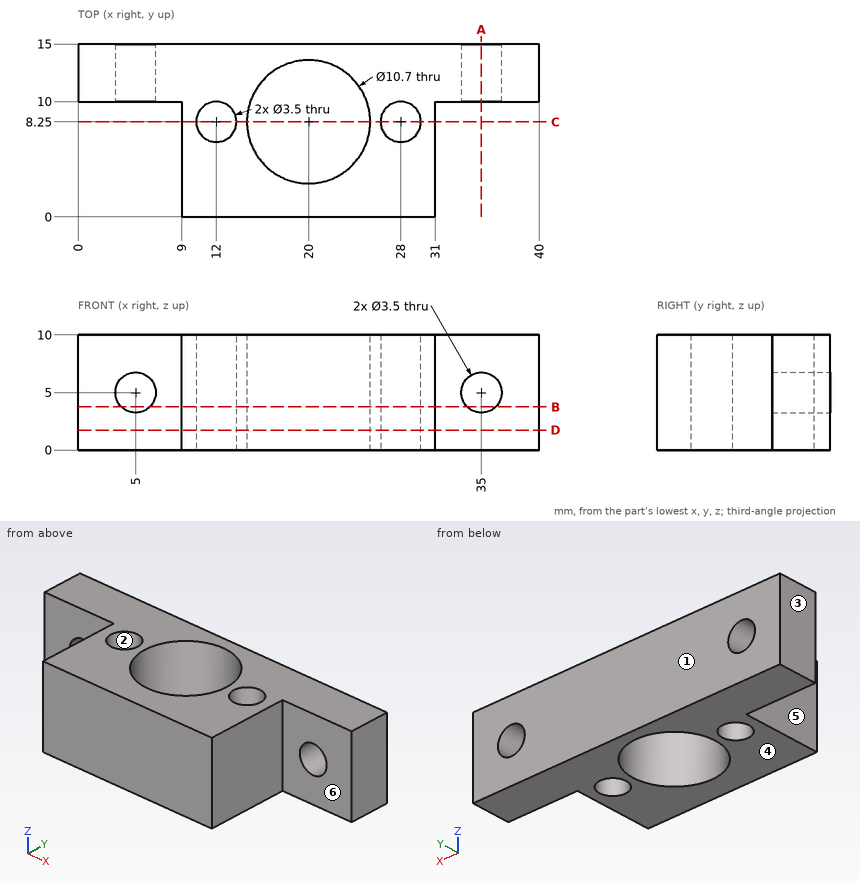
Design review of the part shown in the three views and the two pictorial views. Dimensions are in mm from the part's minimum x, y and z. A direction names the side the tool comes from. Give positions to 0.01 mm unless a question says otherwise; leave off trailing zeros. Write each loop counter-clockwise with the first axis right and the second up, starting at its lowest first coordinate (ties: lowest second). Pieces come first, ordered by that corner, then holes. Notation, with made-up numbers: (-17.75, 30.25) -> (38.25, 30.25) arc R15 ccw to (38.25, 55.25) -> close; hole circle Ø4 at (-8.75, 70). An arc over 180 degrees is marked (long way). Answer in a Markdown table with one row per item.
1) Add section A-A on x = 35. State the section outline as (y, z) points.
Worked answers:
| item | result |
|---|---|
| outline | (10, 0) -> (15, 0) -> (15, 3.25) -> (10, 3.25) -> close; (10, 6.75) -> (15, 6.75) -> (15, 10) -> (10, 10) -> close |
2) Add section D-D on z = 1.75. State the section outline as (x, y) points.
Worked answers:
| item | result |
|---|---|
| outline | (0, 10) -> (9, 10) -> (9, 0) -> (31, 0) -> (31, 10) -> (40, 10) -> (40, 15) -> (0, 15) -> close; hole circle Ø3.5 at (12, 8.25); hole circle Ø10.7 at (20, 8.25); hole circle Ø3.5 at (28, 8.25) |
3) Clearance check with flat-ended pins moving along their axes: P1, Ø2, axis at y = 2, z = 8.5, coming from the -X side; P2, Ø3, axis at y = 4, z = 5.5, coming from the +X side; P3, Ø5.5, axis at x = 35, z = 5, coming from the +Y side; P4, Ø4.5, axis at x = 34.5, z = 4.5, coming from the -Y side. State where each tip first meets the part, or that it passes through.
Worked answers:
| item | result |
|---|---|
| P1 | x = 9 |
| P2 | x = 31 |
| P3 | y = 15 |
| P4 | y = 10 |
4) For L1, parallel to Y at x = 20, z = 6.25; L2, parallel to Y at x = 28, z = 3.25; L3, parallel to Z at x = 5, y = 12.35, list the stretches that pass through material, from the lowest coordinate up. Write a range as [from, to].
Worked answers:
| item | result |
|---|---|
| L1 | [0, 2.9], [13.6, 15] |
| L2 | [0, 6.5], [10, 15] |
| L3 | [0, 3.25], [6.75, 10] |
5) Mouldability with a two-part tool opening along X and no side actions: class the marked faces 1, 2 and 3 as +X half, -X half, draft (parallel to the pull), parting line (faces both ways), or undercut.
Worked answers:
| item | result |
|---|---|
| face 1 | draft |
| face 2 | undercut |
| face 3 | -X half |
6) Tool access review of the marked faces 4, 5 and 6: name each direction out of +Z, -Z, +X, -X, +Y, -Y from which nothing blocks a thin tool from reaching the whole face with its end or side.
Worked answers:
| item | result |
|---|---|
| face 4 | -Z, +X, -X, +Y, -Y |
| face 5 | +Z, -Z, -X, -Y |
| face 6 | +Z, -Z, +X, -Y |
7) Add section B-B on z = 3.75. State the section outline as (x, y) points, plus the area to 3 significant figures.
Worked answers:
| item | result |
|---|---|
| outline | (0, 10) -> (3.78, 10) -> (3.78, 15) -> (0, 15) -> close; (6.22, 10) -> (9, 10) -> (9, 0) -> (31, 0) -> (31, 10) -> (33.78, 10) -> (33.78, 15) -> (6.22, 15) -> close; (36.22, 10) -> (40, 10) -> (40, 15) -> (36.22, 15) -> close; hole circle Ø3.5 at (12, 8.25); hole circle Ø10.7 at (20, 8.25); hole circle Ø3.5 at (28, 8.25) |
| area | 286 mm² |
8) Add section C-C on y = 8.25. State the section outline as (x, z) points.
Worked answers:
| item | result |
|---|---|
| outline | (9, 0) -> (10.25, 0) -> (10.25, 10) -> (9, 10) -> close; (13.75, 0) -> (14.65, 0) -> (14.65, 10) -> (13.75, 10) -> close; (25.35, 0) -> (26.25, 0) -> (26.25, 10) -> (25.35, 10) -> close; (29.75, 0) -> (31, 0) -> (31, 10) -> (29.75, 10) -> close |
